Job drawing, mm, ordinate dimensions from the low corner. One solid piece. A direction names the side the tool comes from. Coordinates: 2 decimals unless noted, no trailing zeros. Loops run counter-clockwise (first coordinate to the right, second up) from the corner with the lowest first, then second, coordinate; pieces in that order, holes last. Notation, with made-up numbers: M 9,17 L 54,17 A24 cw 54,49 Z; hole C 68,10 d10. An arc over 180 degrees is marked long. Answer as a JSON object with one key per item and string values. Group by question number.
1. Saw through at D-D on x = 3.5. Write the cut outline in (y, z), then the cut area to 3 significant figures.
2. Drop flat-ended pins along their axis: pin 1 Ø6 at (x, y) = (12, 3.5) entering from +Z; pin 2 Ø5 at (x, z) = (12.5, 4.5) entering from -Y; pin 3 Ø3 at (x, z) = (6.5, 7.5) entering from -Y (3 decimals). Give the stop position or say it passes through.
3. Drill centre lines: L1, parallel to Z at x = 8.75, y = 3.75; L2, parallel to Y at x = 8, z = 1.5 (3 decimals); L3, parallel to Y at x = 9.5, z = 5.5. Where is each one in solid material? Low to high.
4. Saw through at A-A on y = 8. Write the cut outline in (x, z) (3 decimals).
5. Saw through at C-C on z = 3.5. Write the cut outline in (x, y) (3 decimals).
6. 3-axis set-ups, long thin cutter, end or side, ignore diameter. For the marked faces 1 and 2: which of +Z, -Z, +X, -X, +Y, -Y reach the whole face in a straight line?
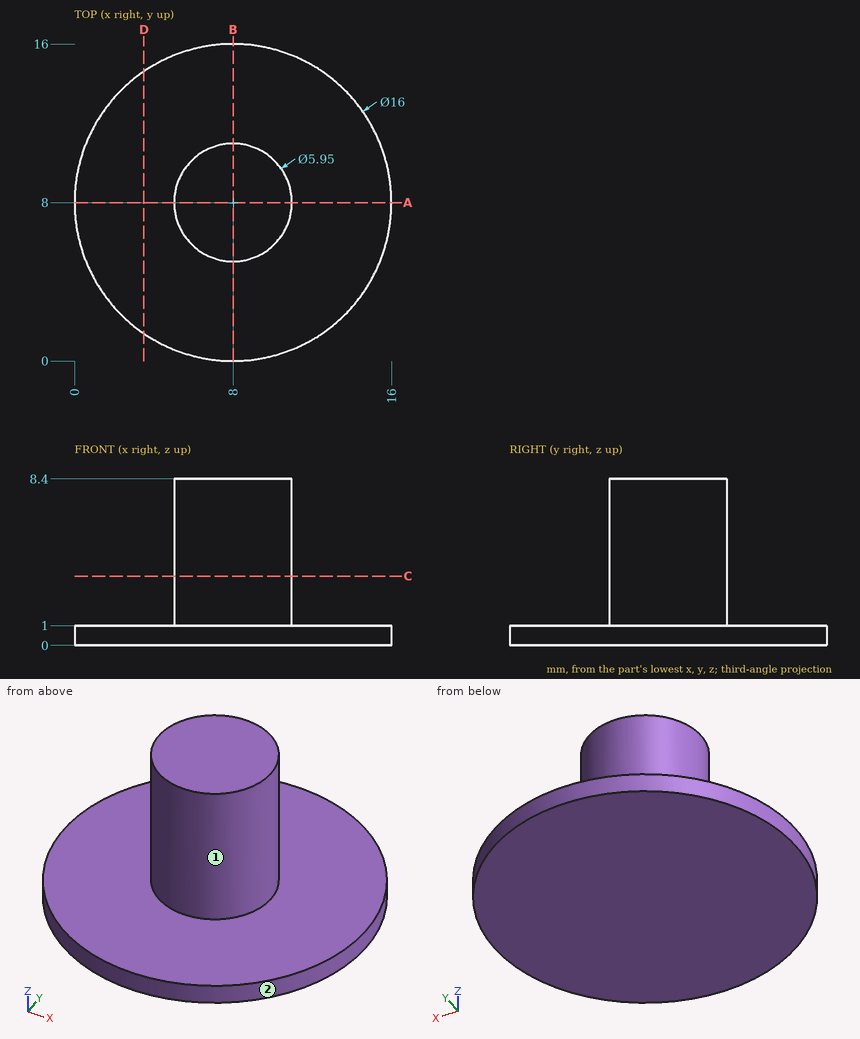
Outcome:
{
 "1": {"outline": "M 1.39,0 L 14.61,0 L 14.61,1 L 1.39,1 Z", "area": "13.2 mm²"},
 "2": {"pin 1": "stops at z = 1", "pin 2": "stops at y = 5.8", "pin 3": "stops at y = 5.025"},
 "3": {"L1": "z = 0 to 1", "L2": "y = 5.025 to 10.975", "L3": "y = 5.43 to 10.57"},
 "4": {"outline": "M 0,0 L 16,0 L 16,1 L 10.975,1 L 10.975,8.4 L 5.025,8.4 L 5.025,1 L 0,1 Z"},
 "5": {"outline": "C 8,8 d5.95"},
 "6": {"face 1": "+Z", "face 2": "+Z, -Z"}
}
